Check sheet for the modelled part. Datum: model origin and axes. Units: mm. Coordinates: 2 decimals unless noted, no trailing zeros. Order: outer loops, then holes, each group sorted by start corner. A loop starts at its lowest first (then second) coordinate and runs counter-clockwise, first axis right, second up. Notation, with made-up numbers: M 22.25,-36 L 80.25,-36 A11 ccw 80.25,-30 Z; hole C -7,-27.5 d7. An arc over 180 degrees is marked long. Answer in a Markdown table with one row per item. Add a question column.
from build123d import *

# Parameters (mm, degrees)
CONG_1_R         = 0.4
D_GAGEMENT_M51_D = 5.3


with BuildPart() as part:
    # Esquisse2 → Révolution1 (revolve)
    with BuildSketch(Plane.XY):
        Polygon((-7, 3), (-5, 0), (-7, -3), (0, -3), (0, 3), align=None)
    revolve(axis=Axis((0, 3, 0), (0, -1, 0)))

    # Congé1
    cong_1_edges = [part.edges().sort_by_distance(p)[0] for p in [
        (7, 3, 0),
        (5, 0, 0),
        (7, -3, 0),
    ]]
    fillet(cong_1_edges, radius=CONG_1_R)

    # Dégagement M51 (through all)
    with Locations(Plane(origin=(0, 3, 0), x_dir=(1, 0, 0), z_dir=(0, 1, 0))):
        with Locations((0, 0)):
            Hole(D_GAGEMENT_M51_D / 2)


solid = part.part
1. Release check for a two-part mould opening along Y. For faces 1 (the flat face through (0, -3, 3)), 2 (the conical face through (-4.84, -0.36, 2.01)), 3 (the flat face through (0, 3, 3)) record: released by +Y, released by -Y, zero draft, split by the parting line, or undercut.
2. Go/stop test with a flat-tipped pin: pin 1 Ø3 at (y, z) = (1.5, 1.5) entering from +X. Record where the tip stops, or that it passes through.
3. Section check A-A on y = 0.6. Enter the section's corners in (x, z), then the cut area to 3 significant figures.
4. Section check B-B on y = -1.85. Enter the section's corners in (x, z), then the cut area to 3 significant figures.
5. Scan lines: line 1 (Z direction, x = 2, y = -1.15); line 2 (Y direction, x = 5.75, z = 2); line 3 (Z direction, x = -0.5, y = -2.5). Record each from-to range of solid material in increasing order.
Result sheet:
| question | item | result |
|---|---|---|
| 1 | face 1 | released by -Y |
| 1 | face 2 | undercut |
| 1 | face 3 | released by +Y |
| 2 | pin 1 | x = 6.64 |
| 3 | outline | C 0,0 d10.8; hole C 0,0 d5.3 |
| 3 | area | 69.5 mm^2 |
| 4 | outline | C 0,0 d12.47; hole C 0,0 d5.3 |
| 4 | area | 100 mm^2 |
| 5 | line 1 | -5.41 to -1.74, 1.74 to 5.41 |
| 5 | line 2 | -3 to -1.63, 1.63 to 3 |
| 5 | line 3 | -6.62 to -2.6, 2.6 to 6.62 |
